Source: CAD feature listing. Evaluate the final solid. Frame: model axes, mm. Give positions to 0.01 mm unless a question says otherwise; leave off trailing zeros. Order: outer loops, then holes, each group sorted by start corner. A loop starts at its lowest first (then second) coordinate and runs counter-clockwise, first axis right, second up. Notation, with made-up numbers: M 48,88 L 88,88 A10 cw 88,101 Z; hole C 58.5,86 d7. An arc over 180 degrees is marked long. Use CSV: the item, a comma, the result in double quotes. Start each with the question number.
1. Section query C-C, the plane y = 83. Return the cut outline in (x, z).
2. Pin query (flat end, axial travel): P1, Ø12, axis at y = 89, z = 685, coming from the +X side; P2, Ø1, axis at y = 91, z = -334, coming from the -X side. Return the tip coordinate at first contact, or that it passes through.
3. Section query A-A, the plane x = 59.5. Return the cut outline in (y, z).
4. Line query: line 1 along Y through (x, z) = (61, -944.5); line 2 along X through (y, z) = (216.5, 287); line 3 along Y through (x, z) = (115.5, 946.5). Output: solid intervals per line, ascending. Write a range as [from, to].
5. Section query B-B, the plane z = -360. Return the cut outline in (x, y), plus the area to 3 significant figures.
from build123d import *

# Parameters (mm, degrees)
BASESTEELW_DEPTH = 1066.8


with BuildPart() as part:
    # Sketch1 → BaseSteelW (new, symmetric)
    with BuildSketch(Plane.XY):
        with BuildLine():
            Line((0, 0), (0, 15.748))
            Line((0, 15.748), (84.709, 15.748))
            ThreePointArc((84.709, 15.748), (93.689256121, 19.467743879), (97.409, 28.448))
            Line((97.409, 28.448), (97.409, 228.092))
            ThreePointArc((97.409, 228.092), (93.689256121, 237.072256121), (84.709, 240.792))
            Line((84.709, 240.792), (0, 240.792))
            Line((0, 240.792), (0, 256.54))
            Line((0, 256.54), (203.708, 256.54))
            Line((203.708, 256.54), (203.708, 240.792))
            Line((203.708, 240.792), (118.999, 240.792))
            ThreePointArc((118.999, 240.792), (110.018743879, 237.072256121), (106.299, 228.092))
            Line((106.299, 228.092), (106.299, 28.448))
            ThreePointArc((106.299, 28.448), (110.018743879, 19.467743879), (118.999, 15.748))
            Line((118.999, 15.748), (203.708, 15.748))
            Line((203.708, 15.748), (203.708, 0))
            Line((203.708, 0), (0, 0))
        make_face()
    extrude(amount=BASESTEELW_DEPTH, both=True)


solid = part.part
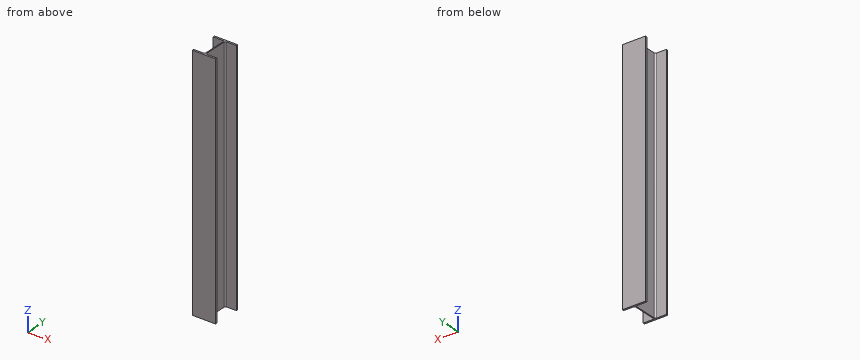
Result set:
1,outline,"M 97.41,-1066.8 L 106.3,-1066.8 L 106.3,1066.8 L 97.41,1066.8 Z"
2,P1,"x = 106.3"
2,P2,"x = 97.41"
3,outline,"M 0,-1066.8 L 15.75,-1066.8 L 15.75,1066.8 L 0,1066.8 Z; M 240.79,-1066.8 L 256.54,-1066.8 L 256.54,1066.8 L 240.79,1066.8 Z"
4,line 1,"[0, 15.75], [240.79, 256.54]"
4,line 2,"[97.41, 106.3]"
4,line 3,"[0, 16.24], [240.3, 256.54]"
5,outline,"M 0,0 L 203.71,0 L 203.71,15.75 L 119,15.75 A12.7 cw 106.3,28.45 L 106.3,228.09 A12.7 cw 119,240.79 L 203.71,240.79 L 203.71,256.54 L 0,256.54 L 0,240.79 L 84.71,240.79 A12.7 cw 97.41,228.09 L 97.41,28.45 A12.7 cw 84.71,15.75 L 0,15.75 Z"
5,area,"8,560 mm2"
